```python
from build123d import *

# Parameters (mm, degrees)
SKETCH1_W           = 103
SKETCH1_H           = 50
BOSS_EXTRUDE1_DEPTH = 2
SKETCH3_R           = 2
CUT_EXTRUDE1_DEPTH  = 7
SKETCH4_R           = 2.5
CUT_EXTRUDE2_DEPTH  = 7
SKETCH6_W           = 43
SKETCH6_H           = 2
BOSS_EXTRUDE3_DEPTH = 100
SKETCH7_R           = 1.5
CUT_EXTRUDE3_DEPTH  = 30


with BuildPart() as part:
    # Sketch1 → Boss-Extrude1 (new body)
    with BuildSketch(Plane.XY):
        Rectangle(SKETCH1_W, SKETCH1_H)
    extrude(amount=BOSS_EXTRUDE1_DEPTH)

    # Sketch3 → Cut-Extrude1 (cut)
    with BuildSketch(Plane.XY.offset(2)):
        with Locations((-11.845, 9)):
            Circle(SKETCH3_R)
        with Locations((-11.845, -9)):
            Circle(SKETCH3_R)
        with Locations((11.845, -9)):
            Circle(SKETCH3_R)
        with Locations((11.845, 9)):
            Circle(SKETCH3_R)
    extrude(amount=-CUT_EXTRUDE1_DEPTH, mode=Mode.SUBTRACT)

    # Sketch4 → Cut-Extrude2 (cut)
    with BuildSketch(Plane.XY.offset(2)):
        with Locations((-36.5, 7.5)):
            Circle(SKETCH4_R)
        with Locations((-36.5, -7.5)):
            Circle(SKETCH4_R)
        with Locations(Location((36.5, -7.5, 0), (0, 0, 180))):
            Circle(SKETCH4_R)
        with Locations(Location((36.5, 7.5, 0), (0, 0, 180))):
            Circle(SKETCH4_R)
    extrude(amount=-CUT_EXTRUDE2_DEPTH, mode=Mode.SUBTRACT)

    # Sketch6 → Boss-Extrude3 (add)
    with BuildSketch(Plane(origin=(0, 25, 0), x_dir=(1, 0, 0), z_dir=(0, 1, 0))):
        with Locations((0, -1)):
            Rectangle(SKETCH6_W, SKETCH6_H)
    extrude(amount=BOSS_EXTRUDE3_DEPTH)

    # Sketch7 → Cut-Extrude3 (cut)
    with BuildSketch(Plane.XY.offset(2)):
        with Locations((0, 112)):
            Circle(SKETCH7_R)
        with Locations((0, 99)):
            Circle(SKETCH7_R)
        with Locations((0, 86)):
            Circle(SKETCH7_R)
        with Locations((0, 73)):
            Circle(SKETCH7_R)
    extrude(amount=-CUT_EXTRUDE3_DEPTH, mode=Mode.SUBTRACT)


solid = part.part
```
The listing builds one solid part. Answer for the finished solid, in the listing's coordinates (mm). Coordinates: 2 decimals unless noted, no trailing zeros. Loops run counter-clockwise (first coordinate to the right, second up) from the corner with the lowest first, then second, coordinate; pieces in that order, holes last. Notation, with made-up numbers: (58.5, 27.5) -> (91.5, 27.5) arc R17 cw to (91.5, 31.5) -> close; hole circle Ø4 at (43, 28.5). An arc over 180 degrees is marked (long way). Use one line per item in the form item = value. Start each with the question number.
Item 1: Consider L1, parallel to Y at x = 0, z = 0.1; L2, parallel to Y at x = 41.5, z = 0.5; L3, parallel to Y at x = -35.5, z = 0.25. Determine where each line is inside the solid, lowest interval first. Write a range as [from, to].
Item 2: The part is cut by section A-A on y = 112. Determine the outline of the cut face in (x, z).
Item 3: The part is cut by section B-B on x = -36.5. Determine the outline of the cut face in (y, z), then the cut area to 3 significant figures.
Item 4: Flat-ended cylindrical pins translate along their axes: pin 1 Ø3 at (x, y) = (-36.5, 7.5) entering from -Z; pin 2 Ø0.6 at (y, z) = (55, 0.5) entering from -X; pin 3 Ø0.6 at (x, z) = (-30.5, 0.5) entering from +Y. Find the tip coordinate at first contact, or state that the pin passes through.
Item 5: The mould has two halves that part along Y. Classify faces 1 (the face through (-0.195, 87.487, 1.014)), 2 (the face through (34.19, 8.46, 1.01)), 3 (the face through (-1, 34, 0)): released by +Y, released by -Y, zero draft, split by the parting line, or undercut.
Item 6: The part is cut by section C-C on z = 0.6. Count the separate pieces of the cut face and the enclosed holes in it, then the cut area to 3 significant figures.
Item 7: The part is cut by section D-D on y = 27. Determine the outline of the cut face in (x, z).
Answer key:
q1.L1 = [-25, 71.5], [74.5, 84.5], [87.5, 97.5], [100.5, 110.5], [113.5, 125]
q1.L2 = [-25, 25]
q1.L3 = [-25, -9.79], [-5.21, 5.21], [9.79, 25]
q2.outline = (-21.5, 0) -> (-1.5, 0) -> (-1.5, 2) -> (-21.5, 2) -> close; (1.5, 0) -> (21.5, 0) -> (21.5, 2) -> (1.5, 2) -> close
q3.outline = (-25, 0) -> (-10, 0) -> (-10, 2) -> (-25, 2) -> close; (-5, 0) -> (5, 0) -> (5, 2) -> (-5, 2) -> close; (10, 0) -> (25, 0) -> (25, 2) -> (10, 2) -> close
q3.area = 80.0 mm2
q4.pin_1 = through
q4.pin_2 = -21.5
q4.pin_3 = 25
q5.face_1 = undercut
q5.face_2 = undercut
q5.face_3 = zero draft
q6.separate_pieces = 1
q6.enclosed_holes = 12
q6.area = 9,290 mm2
q7.outline = (-21.5, 0) -> (21.5, 0) -> (21.5, 2) -> (-21.5, 2) -> close
